Could you check a few things on this model? Use its own coordinates, in mm. Face numbers are marked on the shaded views. A direction names the side the tool comes from. Round coordinates to 2 decimals unless told otherwise and drop trailing zeros. Write each loop counter-clockwise with the first axis right and the second up, starting at its lowest first coordinate (ties: lowest second). Pieces come first, ordered by that corner, then holes. Notation, with made-up numbers: (20, 3.5) -> (31, 3.5) arc R20 cw to (31, 18.5) -> close; hole circle Ø4 at (67.5, -0.5). An arc over 180 degrees is marked (long way). Answer in a Markdown table with one row per item.
from build123d import *

# Parameters (mm, degrees)
SKETCH1_W           = 130
SKETCH1_H           = 40
BOSS_EXTRUDE1_DEPTH = 10
SKETCH3_W           = 31
SKETCH3_H           = 31
BOSS_EXTRUDE3_DEPTH = 50
SKETCH4_W           = 29
SKETCH4_H           = 48
CUT_EXTRUDE1_DEPTH  = 90.360226052
CUT_EXTRUDE2_REACH  = 92.692
SKETCH5_R           = 2.5
SKETCH2_W           = 15
SKETCH2_H           = 100
BOSS_EXTRUDE4_DEPTH = 20
SKETCH6_R           = 5
CUT_EXTRUDE3_DEPTH  = 20


with BuildPart() as part:
    # Sketch1 → Boss-Extrude1 (new body)
    with BuildSketch(Plane(origin=(0, 0, 0), x_dir=(1, 0, 0), z_dir=(0, 1, 0))):
        Rectangle(SKETCH1_W, SKETCH1_H)
    extrude(amount=BOSS_EXTRUDE1_DEPTH)

    # Sketch3 → Boss-Extrude3 (add)
    with BuildSketch(Plane.XZ):
        Rectangle(SKETCH3_W, SKETCH3_H)
    extrude(amount=BOSS_EXTRUDE3_DEPTH)

    # Sketch4 → Cut-Extrude1 (cut, through all)
    with BuildSketch(Plane(origin=(0, 0, -15.5), x_dir=(-1, 0, 0), z_dir=(0, 0, -1))):
        with Locations((0, -25)):
            Rectangle(SKETCH4_W, SKETCH4_H)
    extrude(amount=-CUT_EXTRUDE1_DEPTH, mode=Mode.SUBTRACT)

    # Sketch5 → Cut-Extrude2 (cut, up to next)
    with BuildSketch(Plane.XZ.offset(50), mode=Mode.PRIVATE) as cut_extrude2_sk1:
        with Locations(Location((0, 0, 0), (0, 0, 270))):
            Circle(SKETCH5_R)
    cut_extrude2_tool1 = extrude(cut_extrude2_sk1.sketch, amount=-CUT_EXTRUDE2_REACH, mode=Mode.PRIVATE) & part.part
    add(cut_extrude2_tool1.solids().sort_by_distance((0, -50, 0))[0], mode=Mode.SUBTRACT)

    # Sketch2 → Boss-Extrude4 (add)
    with BuildSketch(Plane(origin=(0, 10, 0), x_dir=(1, 0, 0), z_dir=(0, 1, 0))):
        with Locations((-57.5, 0)):
            Rectangle(SKETCH2_W, SKETCH2_H)
    boss_extrude4 = extrude(amount=BOSS_EXTRUDE4_DEPTH)

    # Sketch6 → Cut-Extrude3 (cut)
    with BuildSketch(Plane(origin=(-50, 0, 0), x_dir=(0, 0, -1), z_dir=(1, 0, 0))):
        with Locations((-40, 19.678033473)):
            Circle(SKETCH6_R)
        with Locations((40, 19.678033473)):
            Circle(SKETCH6_R)
    cut_extrude3 = extrude(amount=-CUT_EXTRUDE3_DEPTH, mode=Mode.SUBTRACT)

    # Mirror1: Boss-Extrude4, Cut-Extrude3 across plane
    add(boss_extrude4.mirror(Plane(origin=(0, 0, 0), x_dir=(0, 0, 1), z_dir=(1, 0, 0))))
    add(cut_extrude3.mirror(Plane(origin=(0, 0, 0), x_dir=(0, 0, 1), z_dir=(1, 0, 0))), mode=Mode.SUBTRACT)


solid = part.part
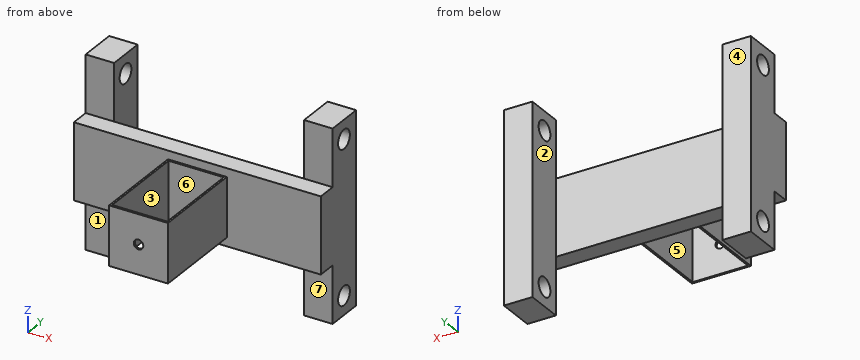
1) Imagine slicing it at C-C, the plane z = -7. Please give me the cut outline in (x, y), plus the area to 3 significant figures.
Findings:
| item | result |
|---|---|
| outline | (-65, 0) -> (-15.5, 0) -> (-15.5, -50) -> (15.5, -50) -> (15.5, 0) -> (65, 0) -> (65, 30) -> (50, 30) -> (50, 10) -> (-50, 10) -> (-50, 30) -> (-65, 30) -> close; hole (-14.5, -49) -> (14.5, -49) -> (14.5, -1) -> (-14.5, -1) -> close |
| area | 2,060 mm^2 |
2) For pin 1 (3 mm diameter, centred on x = 0, z = 0, fed in from +Y); pin 2 (1.5 mm diameter, centred on x = 32.5, z = -5.5, fed in from -Y); pin 3 (12 mm diameter, centred on x = 57, z = -40, fed in from -Y); pin 4 (16 mm diameter, centred on y = 19.68, z = 40, fed in from +X), each with a flat end and sliding along its axis, tell me the tip position at first contact or that it passes through.
Findings:
| item | result |
|---|---|
| pin 1 | stops at y = 10 |
| pin 2 | stops at y = 0 |
| pin 3 | stops at y = 10 |
| pin 4 | stops at x = 65 |
3) Thinking about a two-plate mould opening in Y: for the marked faces 4, 5, 6 and 7, which applies, +Y half, -Y half, draft (parallel to the pull), parting line (faces both ways), or undercut?
Findings:
| item | result |
|---|---|
| face 4 | +Y half |
| face 5 | undercut |
| face 6 | undercut |
| face 7 | -Y half |
4) Imagine slicing it at A-A, the plane z = 26. Please give me the cut outline in (x, y), plus the area to 3 significant figures.
Findings:
| item | result |
|---|---|
| outline | (-65, 10) -> (-50, 10) -> (-50, 30) -> (-65, 30) -> close; (50, 10) -> (65, 10) -> (65, 30) -> (50, 30) -> close |
| area | 600 mm^2 |
5) Imagine slicing it at B-B, the plane x = 0. Please give me the cut outline in (y, z).
Findings:
| item | result |
|---|---|
| outline | (-50, -15.5) -> (-49, -15.5) -> (-49, -2.5) -> (-50, -2.5) -> close; (-50, 2.5) -> (-49, 2.5) -> (-49, 15.5) -> (-50, 15.5) -> close; (-1, -15.5) -> (0, -15.5) -> (0, -20) -> (10, -20) -> (10, 20) -> (0, 20) -> (0, 15.5) -> (-1, 15.5) -> close |
6) For the marked faces 1, 2 and 3, which set-ups out of +Z, -Z, +X, -X, +Y, -Y let a thin tool reach every point of the face, with its end or its side?
Findings:
| item | result |
|---|---|
| face 1 | -Z, +X, -X, -Y |
| face 2 | +Z, -Z, +Y |
| face 3 | +Z, -Z |
7) Please list where these lines run through material, in increasing order: line 1 (X direction, y = 15, z = -3); line 2 (X direction, y = -27, z = 4); line 3 (Y direction, x = -55, z = 40).
Findings:
| item | result |
|---|---|
| line 1 | x = -65 to -50, 50 to 65 |
| line 2 | x = -15.5 to -14.5, 14.5 to 15.5 |
| line 3 | y = 10 to 14.68, 24.68 to 30 |
8) Imagine slicing it at D-D, the plane z = 40. Please give me the cut outline in (x, y), plus the area to 3 significant figures.
Findings:
| item | result |
|---|---|
| outline | (-65, 10) -> (-50, 10) -> (-50, 14.68) -> (-65, 14.68) -> close; (-65, 24.68) -> (-50, 24.68) -> (-50, 30) -> (-65, 30) -> close; (50, 10) -> (65, 10) -> (65, 14.68) -> (50, 14.68) -> close; (50, 24.68) -> (65, 24.68) -> (65, 30) -> (50, 30) -> close |
| area | 300 mm^2 |
